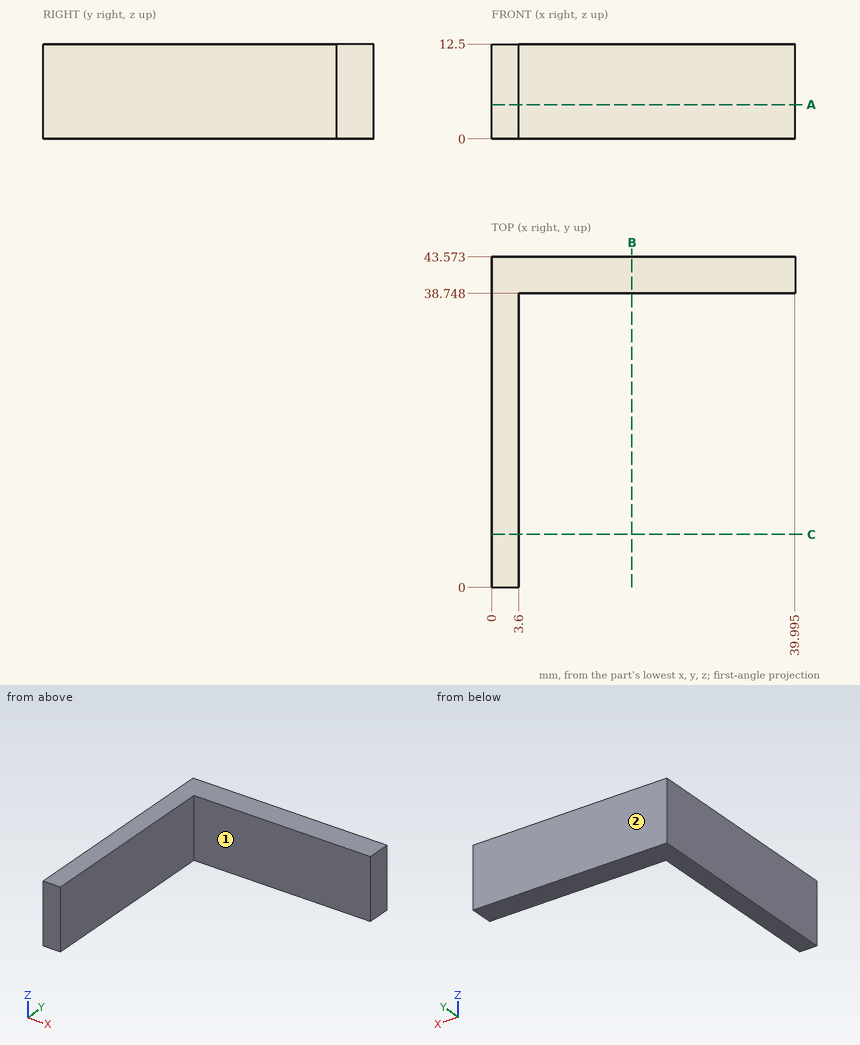
Input: dimensioned drawing with shaded views. Units: mm. Origin: part minimum x, y, z. A direction names the side the tool comes from. Round coordinates to 2 decimals unless told otherwise and drop trailing zeros. Write each loop counter-clockwise with the first axis right and the second up, starting at its lowest first coordinate (ties: lowest second). Pieces come first, ordered by that corner, then holes. Notation, with made-up numbers: (-20, 81.25) -> (28, 81.25) arc R9 cw to (28, 94.25) -> close; hole circle Ø2 at (30, 22). An arc over 180 degrees is marked (long way). Use CSV: the item, a comma, the result in double quotes. Start each with the question number.
Q1. Line query: L1, parallel to Y at x = 33, z = 6.25; L2, parallel to X at y = 5, z = 3.75. Output: solid intervals per line, ascending.
Q2. Section C-C (y = 7). Return loops of the section in (x, z), plus the area to 3 significant figures.
Q3. Section A-A (z = 4.5). Return loops of the section in (x, y) (1 decimal).
Q4. First-contact query: pin 1 Ø6 at (y, z) = (28, 7.5) entering from +X. Flat tip, straight axial feed; report the tip coordinate or a pass-through.
Q5. Section B-B (x = 18.5). Return loops of the section in (y, z).
Q6. Reachability of the marked faces 1 and 2 from +Z, -Z, +X, -X, +Y, -Y: full face, straight path, thin tool, end or side. Return the list, or none.
Result sheet:
1,L1,"38.75 to 43.57"
1,L2,"0 to 3.6"
2,outline,"(0, 0) -> (3.6, 0) -> (3.6, 12.5) -> (0, 12.5) -> close"
2,area,"45.0 mm²"
3,outline,"(0, 0) -> (3.6, 0) -> (3.6, 38.7) -> (40, 38.7) -> (40, 43.6) -> (0, 43.6) -> close"
4,pin 1,"x = 3.6"
5,outline,"(38.75, 0) -> (43.57, 0) -> (43.57, 12.5) -> (38.75, 12.5) -> close"
6,face 1,"+Z, -Z, +X, -Y"
6,face 2,"+Z, -Z, +X, -X, +Y"
